from build123d import *

# Parameters (mm, degrees)
SKETCH1_R             = 95
BOSS_EXTRUDE1_DEPTH   = 9
SKETCH2_R             = 15
CUT_EXTRUDE1_DEPTH    = 135.651401775
SKETCH3_R             = 3.107652879
CUT_EXTRUDE2_DEPTH    = 7.045424
CIRPATTERN1_START     = 1.954576325
CIRPATTERN1_OUTLINE_R = 3.107652879
CIRPATTERN1_DEPTH     = 7.045423675


# Read off the part's stored shape, not the designer's step: CirPattern1
with BuildPart() as part:
    # Sketch1 → Boss-Extrude1 (new body)
    with BuildSketch(Plane(origin=(0, 0, 0), x_dir=(1, 0, 0), z_dir=(0, 1, 0))):
        with Locations(Location((0, 0, 0), (0, 0, 270))):
            Circle(SKETCH1_R)
    extrude(amount=BOSS_EXTRUDE1_DEPTH)

    # Sketch2 → Cut-Extrude1 (cut, through all)
    with BuildSketch(Plane(origin=(0, 0, 0), x_dir=(1, 0, 0), z_dir=(0, 1, 0))):
        with Locations(Location((0, 0, 0), (0, 0, 270))):
            Circle(SKETCH2_R)
    extrude(amount=CUT_EXTRUDE1_DEPTH, mode=Mode.SUBTRACT)

    # Sketch3 → Cut-Extrude2 (cut)
    with BuildSketch(Plane(origin=(0, 9, 0), x_dir=(1, 0, 0), z_dir=(0, 1, 0))):
        with Locations(Location((-33.15170901, 0, 0), (0, 0, 270))):
            Circle(SKETCH3_R)
    extrude(amount=-CUT_EXTRUDE2_DEPTH, mode=Mode.SUBTRACT)

    # CirPattern1 outline → CirPattern1 (cut)
    with BuildSketch(Plane(origin=(0, 0, 0), x_dir=(1, 0, 0), z_dir=(0, 1, 0)).offset(CIRPATTERN1_START)):
        with Locations((-23.441798249, -23.441798249)):
            Circle(CIRPATTERN1_OUTLINE_R)
        with Locations((-23.441798249, 23.441798249)):
            Circle(CIRPATTERN1_OUTLINE_R)
        with Locations((0, 33.15170901)):
            Circle(CIRPATTERN1_OUTLINE_R)
        with Locations((23.441798249, 23.441798249)):
            Circle(CIRPATTERN1_OUTLINE_R)
        with Locations((33.15170901, 0)):
            Circle(CIRPATTERN1_OUTLINE_R)
        with Locations((23.441798249, -23.441798249)):
            Circle(CIRPATTERN1_OUTLINE_R)
        with Locations((0, -33.15170901)):
            Circle(CIRPATTERN1_OUTLINE_R)
    extrude(amount=CIRPATTERN1_DEPTH, mode=Mode.SUBTRACT)


solid = part.part
CAD build for the part. Positions are in the model's coordinates, mm. A direction names the side the tool comes from. Give positions to 0.01 mm unless a question says otherwise; leave off trailing zeros. Order: outer loops, then holes, each group sorted by start corner. A loop starts at its lowest first (then second) coordinate and runs counter-clockwise, first axis right, second up. Notation, with made-up numbers: (69, 68) - (114, 68) arc R25 ccw to (114, 101) - close; hole circle Ø9 at (21, -8). An arc over 180 degrees is marked (long way). Answer in a Markdown table with one row per item.
1. Saw through at D-D, the plane x = 54. Give the cut face in (y, z).
Data:
| item | result |
|---|---|
| outline | (0, -78.16) - (9, -78.16) - (9, 78.16) - (0, 78.16) - close |
2. Saw through at C-C, the plane y = 4.25. Count the separate pieces of the cut face and the enclosed holes in it, plus the area to 3 significant figures.
Data:
| item | result |
|---|---|
| separate pieces | 1 |
| enclosed holes | 9 |
| area | 27,400 mm² |
3. Saw through at B-B, the plane z = 0. Give the cut face in (x, y), plus the area to 3 significant figures.
Data:
| item | result |
|---|---|
| outline | (-95, 0) - (-15, 0) - (-15, 9) - (-30.04, 9) - (-30.04, 1.95) - (-36.26, 1.95) - (-36.26, 9) - (-95, 9) - close; (15, 0) - (95, 0) - (95, 9) - (36.26, 9) - (36.26, 1.95) - (30.04, 1.95) - (30.04, 9) - (15, 9) - close |
| area | 1,350 mm² |
4. Tool access for faces 1 (the cylindrical face through (0.66, 4.437, -14.985)), 2 (the flat face through (33, 1.955, 0)): list every direction of +Z, -Z, +X, -X, +Y, -Y with a clear straight run to the whole face (end or side of a thin tool).
Data:
| item | result |
|---|---|
| face 1 | +Y, -Y |
| face 2 | +Y |
5. Probe probe 1 along X at (y, z) = (6.5, 0); probe 2 along Z at (x, y) = (22, 6.5); probe 3 along Z at (x, y) = (2, 3.5). List the from-to ranges inside material, lowest first. Write a range as [from, to].
Data:
| item | result |
|---|---|
| probe 1 | x = [-95, -36.26], [-30.04, -15], [15, 30.04], [36.26, 95] |
| probe 2 | z = [-92.42, -26.19], [-20.69, 20.69], [26.19, 92.42] |
| probe 3 | z = [-94.98, -35.53], [-30.77, -14.87], [14.87, 30.77], [35.53, 94.98] |
6. Saw through at A-A, the plane x = 0. Give the cut face in (y, z), plus the area to 3 significant figures.
Data:
| item | result |
|---|---|
| outline | (0, -95) - (9, -95) - (9, -36.26) - (1.95, -36.26) - (1.95, -30.04) - (9, -30.04) - (9, -15) - (0, -15) - close; (0, 15) - (9, 15) - (9, 30.04) - (1.95, 30.04) - (1.95, 36.26) - (9, 36.26) - (9, 95) - (0, 95) - close |
| area | 1,350 mm² |
7. Pull direction X, two halves, no side cores. Call faces 3 (the cylindrical face through (22.8, 5.4, -20.4)), 4 (the flat face through (1, 0, 20)), 5 (the cylindrical face through (-92.74, 4.44, -20.59)): pulls with the +X half, pulls with the -X half, needs draft (parallel to the pull), parting line crosses it, or undercut.
Data:
| item | result |
|---|---|
| face 3 | undercut |
| face 4 | needs draft |
| face 5 | parting line crosses it |
8. Flat gauge pins, fed straight in: pin 1 (2 mm diameter, centred on x = -56.5, y = 3.5, fed in from -Z); pin 2 (3.5 mm diameter, centred on x = 23.44, z = -23.44, fed in from +Y); pin 3 (3 mm diameter, centred on x = 26.5, y = 5, fed in from -Z); pin 4 (18 mm diameter, centred on x = 0, z = 0, fed in from -Y). Where does each tip first touch, or does it go through?
Data:
| item | result |
|---|---|
| pin 1 | stops at z = -77.1 |
| pin 2 | stops at y = 1.95 |
| pin 3 | stops at z = -91.65 |
| pin 4 | passes through |
